Could you check a few things on this model? Use its own coordinates, in mm. A direction names the side the tool comes from. Coordinates: 2 decimals unless noted, no trailing zeros. Loops run counter-clockwise (first coordinate to the right, second up) from the corner with the lowest first, then second, coordinate; pieces in that order, holes last. Notation, with made-up numbers: M 61.25,72.25 L 88.25,72.25 A24 cw 88.25,94.25 Z; hole C 63,0 d2. An arc over 180 degrees is marked long. Return JSON: item names as keys, results as strings. Group by question number.
from build123d import *

# Parameters (mm, degrees)
SKETCH_1_R          = 36
SKETCH_1_R_2        = 1.5
EXTRUDE_1_DEPTH     = 41
SKETCH_2_R          = 3
CUT_EXTRUDE_1_DEPTH = 12
SKETCH_3_R          = 4
CUT_EXTRUDE_2_DEPTH = 12
SKETCH_4_R          = 1.25
CUT_EXTRUDE_3_DEPTH = 12
CUT_EXTRUDE_START   = -21
SKETCH_5_R          = 36
SKETCH_5_R_2        = 35
CUT_EXTRUDE_4_DEPTH = 21


with BuildPart() as part:
    # 草图1 → 凸台-拉伸1 (new body)
    with BuildSketch(Plane.XY):
        Circle(SKETCH_1_R)
        with Locations((32, 0)):
            Circle(SKETCH_1_R_2, mode=Mode.SUBTRACT)
        with Locations((27.712812921, -16)):
            Circle(SKETCH_1_R_2, mode=Mode.SUBTRACT)
        with Locations((16, -27.712812921)):
            Circle(SKETCH_1_R_2, mode=Mode.SUBTRACT)
        with Locations((0, -32)):
            Circle(SKETCH_1_R_2, mode=Mode.SUBTRACT)
        with Locations((-16, -27.712812921)):
            Circle(SKETCH_1_R_2, mode=Mode.SUBTRACT)
        with Locations((-27.712812921, -16)):
            Circle(SKETCH_1_R_2, mode=Mode.SUBTRACT)
        with Locations((-32, 0)):
            Circle(SKETCH_1_R_2, mode=Mode.SUBTRACT)
        with Locations((-27.712812921, 16)):
            Circle(SKETCH_1_R_2, mode=Mode.SUBTRACT)
        with Locations((-16, 27.712812921)):
            Circle(SKETCH_1_R_2, mode=Mode.SUBTRACT)
        with Locations((0, 32)):
            Circle(SKETCH_1_R_2, mode=Mode.SUBTRACT)
        with Locations((16, 27.712812921)):
            Circle(SKETCH_1_R_2, mode=Mode.SUBTRACT)
        with Locations((27.712812921, 16)):
            Circle(SKETCH_1_R_2, mode=Mode.SUBTRACT)
    extrude(amount=EXTRUDE_1_DEPTH)

    # 草图2 → 切除-拉伸1 (cut)
    with BuildSketch(Plane.XY.offset(41)):
        with Locations((16, 0)):
            Circle(SKETCH_2_R)
        with Locations((11.313708499, -11.313708499)):
            Circle(SKETCH_2_R)
        with Locations((0, -16)):
            Circle(SKETCH_2_R)
        with Locations((-11.313708499, -11.313708499)):
            Circle(SKETCH_2_R)
        with Locations((-16, 0)):
            Circle(SKETCH_2_R)
        with Locations((-11.313708499, 11.313708499)):
            Circle(SKETCH_2_R)
        with Locations((0, 16)):
            Circle(SKETCH_2_R)
        with Locations((11.313708499, 11.313708499)):
            Circle(SKETCH_2_R)
    extrude(amount=-CUT_EXTRUDE_1_DEPTH, mode=Mode.SUBTRACT)

    # 草图3 → 切除-拉伸2 (cut)
    with BuildSketch(Plane(origin=(0, 0, 0), x_dir=(-1, 0, 0), z_dir=(0, 0, -1))):
        Circle(SKETCH_3_R)
    extrude(amount=-CUT_EXTRUDE_2_DEPTH, mode=Mode.SUBTRACT)

    # 草图4 → 切除-拉伸3 (cut)
    with BuildSketch(Plane(origin=(0, 0, 0), x_dir=(-1, 0, 0), z_dir=(0, 0, -1))):
        with Locations((7, 0)):
            Circle(SKETCH_4_R)
        with Locations((0, -7)):
            Circle(SKETCH_4_R)
        with Locations((-7, 0)):
            Circle(SKETCH_4_R)
        with Locations((0, 7)):
            Circle(SKETCH_4_R)
    extrude(amount=-CUT_EXTRUDE_3_DEPTH, mode=Mode.SUBTRACT)

    # 草图5 → 切除-拉伸4 (cut)
    with BuildSketch(Plane.XY.offset(41).offset(CUT_EXTRUDE_START)):
        Circle(SKETCH_5_R)
        Circle(SKETCH_5_R_2, mode=Mode.SUBTRACT)
    extrude(amount=CUT_EXTRUDE_4_DEPTH, mode=Mode.SUBTRACT)


solid = part.part
(1) Will these pins go through, and if not, where does the flat tip stop? P1, Ø1, axis at x = -19, z = 10, coming from the -Y side; P2, Ø12, axis at x = -22.5, z = 31, coming from the +Y side; P3, Ø1.8, axis at x = -16, y = -27.71, coming from the -Z side; P4, Ø2.5, axis at x = 1.5, y = -0.5, coming from the -Z side.
(2) Imagine slicing it at B-B, the plane y = 0. Count the separate pieces of the cut face and the enclosed holes in it, then the cut area to 3 significant figures.
(3) Imagine slicing it at A-A, the plane x = 32. Write out the boundary of the cut face in (y, z).
(4) If I drill on L1, parallel to Y at x = 0, z = 5; L2, parallel to X at y = -9.5, z = 29.5; L3, parallel to Y at x = -16, z = 34.5, over which ranges is the centre line in solid material (lowest first)? Write a range as [from, to].
(5) For faces 1 (the face through (-33.2, -0.9, 20.2)), 2 (the face through (11, 11, 29)), 3 (the face through (8.25, 0.05, 5.92)), which set-ups out of +Z, -Z, +X, -X, +Y, -Y let a thin tool reach every point of the face, with its end or its side?
(6) We'd pull the mould along Y, two halves only. Please class faces 4 (the face through (-9, 1, 0)), 5 (the face through (-4.686, 35.694, 9.86)), 6 (the face through (-17.106, -26.699, 20.213)): +Y half, -Y half, draft (parallel to the pull), parting line (faces both ways), or undercut.
(7) Imagine slicing it at C-C, the plane x = -15.5. Write out the boundary of the cut face in (y, z).
Checks:
{
 "1": {"P1": "y = -30.88", "P2": "y = 30.87", "P3": "through", "P4": "z = 12"},
 "2": {"separate pieces": "3", "enclosed holes": "0", "area": "2,360 mm²"},
 "3": {"outline": "M -16.49,0 L -1.5,0 L -1.5,41 L -14.18,41 L -14.18,20 L -16.49,20 Z; M 1.5,0 L 16.49,0 L 16.49,20 L 14.18,20 L 14.18,41 L 1.5,41 Z"},
 "4": {"L1": "[-36, -33.5], [-30.5, -8.25], [-5.75, -4], [4, 5.75], [8.25, 30.5], [33.5, 36]", "L2": "[-33.69, -13.7], [-8.92, 8.92], [13.7, 33.69]", "L3": "[-31.13, -29.21], [-26.21, -3], [3, 26.21], [29.21, 31.13]"},
 "5": {"face 1": "+Z, -Z", "face 2": "+Z", "face 3": "-Z"},
 "6": {"face 4": "draft", "face 5": "parting line", "face 6": "undercut"},
 "7": {"outline": "M -32.49,0 L -29.13,0 L -29.13,41 L -31.38,41 L -31.38,20 L -32.49,20 Z; M -26.3,0 L 26.3,0 L 26.3,41 L 2.96,41 L 2.96,29 L -2.96,29 L -2.96,41 L -26.3,41 Z; M 29.13,0 L 32.49,0 L 32.49,20 L 31.38,20 L 31.38,41 L 29.13,41 Z"}
}
